Here's how the part is built. I have some questions about the finished solid (model axes, mm). Face numbers are marked on the shaded views. A direction names the side the tool comes from. Round coordinates to 2 decimals unless told otherwise and drop trailing zeros. Order: outer loops, then holes, each group sorted by start corner. A loop starts at its lowest first (then second) coordinate and runs counter-clockwise, first axis right, second up.
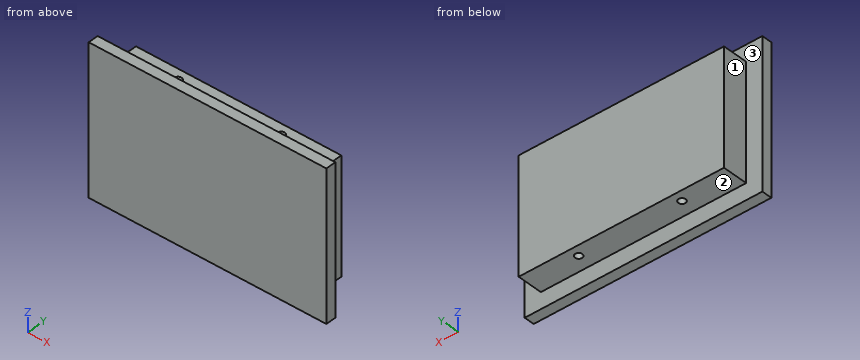
```python
from build123d import *

# Parameters (mm, degrees)
MAIN_SKETCH_W                         = 73.5
MAIN_SKETCH_H                         = 45.5
MAIN_SKETCH_W_2                       = 63.5
MAIN_SKETCH_H_2                       = 35.5
LIP_DEPTH                             = 3.175
MOUNTING_BASE_OUTLINE_W               = 63.5
MOUNTING_BASE_OUTLINE_H               = 35.5
MOUNTING_BASE_DEPTH                   = 11
HEATER_CART_4_40_TAPS_D               = 2.2606
HEATER_CART_4_40_TAPS_DEPTH           = 7.595
HEATER_CART_4_40_TAPS_TIP             = 0.679152758
HEATER_CART_4_40_TAPS_ON_FACE_2_D     = 2.2606
HEATER_CART_4_40_TAPS_ON_FACE_2_DEPTH = 7.595
HEATER_CART_4_40_TAPS_ON_FACE_2_TIP   = 0.679152758


# Read off the part's stored shape, not the designer's step: Mounting_Base
with BuildPart() as part:
    # Main_Sketch → Lip (new body)
    with BuildSketch(Plane(origin=(0, 0, 0), x_dir=(1, 0, 0), z_dir=(0, 1, 0))):
        with Locations((36.75, -22.75)):
            Rectangle(MAIN_SKETCH_W, MAIN_SKETCH_H)
        with Locations((36.75, -22.75)):
            Rectangle(MAIN_SKETCH_W_2, MAIN_SKETCH_H_2, mode=Mode.SUBTRACT)
    extrude(amount=LIP_DEPTH)

    # Mounting_Base outline → Mounting_Base (add)
    with BuildSketch(Plane(origin=(0, 0, 0), x_dir=(1, 0, 0), z_dir=(0, 1, 0))):
        with Locations((36.75, -22.75)):
            Rectangle(MOUNTING_BASE_OUTLINE_W, MOUNTING_BASE_OUTLINE_H)
    extrude(amount=MOUNTING_BASE_DEPTH)

    # Heater_Cart_#4-40_Taps
    with Locations(Plane(origin=(52.725, 7.825, 5), x_dir=(-1, 0, 0), z_dir=(0, 0, -1))):
        with Locations((0, 0), (31.95, 0)):
            Hole(HEATER_CART_4_40_TAPS_D / 2, depth=HEATER_CART_4_40_TAPS_DEPTH)
            with Locations((0, 0, -(HEATER_CART_4_40_TAPS_DEPTH + HEATER_CART_4_40_TAPS_TIP / 2))):  # 118° drill point
                Cone(0, HEATER_CART_4_40_TAPS_D / 2, HEATER_CART_4_40_TAPS_TIP, mode=Mode.SUBTRACT)

    # Heater_Cart_#4-40_Taps on face 2
    with Locations(Plane(origin=(20.775, 7.825, 40.5), x_dir=(1, 0, 0), z_dir=(0, 0, 1))):
        with Locations((0, 0), (31.95, 0)):
            Hole(HEATER_CART_4_40_TAPS_ON_FACE_2_D / 2, depth=HEATER_CART_4_40_TAPS_ON_FACE_2_DEPTH)
            with Locations((0, 0, -(HEATER_CART_4_40_TAPS_ON_FACE_2_DEPTH + HEATER_CART_4_40_TAPS_ON_FACE_2_TIP / 2))):  # 118° drill point
                Cone(0, HEATER_CART_4_40_TAPS_ON_FACE_2_D / 2, HEATER_CART_4_40_TAPS_ON_FACE_2_TIP, mode=Mode.SUBTRACT)


solid = part.part
```
1. I'm going to push flat-ended pins straight in: P1, Ø2.5, axis at y = 5.5, z = 31, coming from the -X side; P2, Ø2, axis at y = 5, z = 36, coming from the +X side; P3, Ø6, axis at x = 11, y = 9, coming from the -Z side. Where does each tip first touch, or does it pass through?
Evaluation:
P1: stops at x = 5
P2: stops at x = 68.5
P3: stops at z = 5
2. If we section it at D-D, the plane y = 4.5: Write out the boundary of the cut face in (x, z), and give its area (3 significant figures).
Evaluation:
outline: (5, 5) - (68.5, 5) - (68.5, 40.5) - (5, 40.5) - close
area: 2,250 mm2
3. If we section it at C-C, the plane z = 10: Write out the boundary of the cut face in (x, y) (3 decimals).
Evaluation:
outline: (0, 0) - (73.5, 0) - (73.5, 3.175) - (68.5, 3.175) - (68.5, 11) - (5, 11) - (5, 3.175) - (0, 3.175) - close; hole circle Ø2.261 at (20.775, 7.825); hole circle Ø2.261 at (52.725, 7.825)
4. If we section it at B-B, the plane z = 26: Write out the boundary of the cut face in (x, y) (3 decimals).
Evaluation:
outline: (0, 0) - (73.5, 0) - (73.5, 3.175) - (68.5, 3.175) - (68.5, 11) - (5, 11) - (5, 3.175) - (0, 3.175) - close
5. I need wall thicknesses on probe 1 along X at (y, z) = (7.75, 6); probe 2 along X at (y, z) = (8.5, 9.5); probe 3 along X at (y, z) = (5.5, 15). Which ranges of each line are inside material? Lowest first, please.
Evaluation:
probe 1: x = 5 to 19.65, 21.9 to 51.6, 53.85 to 68.5
probe 2: x = 5 to 19.87, 21.68 to 51.82, 53.63 to 68.5
probe 3: x = 5 to 68.5
6. If we section it at A-A, the plane x = 8: Write out the boundary of the cut face in (y, z) (3 decimals), and give its area (3 significant figures).
Evaluation:
outline: (0, 0) - (3.175, 0) - (3.175, 5) - (11, 5) - (11, 40.5) - (3.175, 40.5) - (3.175, 45.5) - (0, 45.5) - close
area: 422 mm2
7. On a 3-axis mill with a long thin cutter (end or side, diameter ignored), from which of +Z, -Z, +X, -X, +Y, -Y can I reach the whole of each face in a straight line? I mean the marked faces 1, 2 and 3. Say none if no direction works.
Evaluation:
face 1: +Z, -Z, -X, +Y
face 2: -Z, +X, -X, +Y
face 3: +Y
